from build123d import *

# Parameters (mm, degrees)
SKETCH1_R                          = 61.976
BOSS_EXTRUDE1_DEPTH                = 1.5875
F_1_4_0_25_DIAMETER_HOLE1_D        = 6.35
F_5_16_0_3125_DIAMETER_HOLE1_D     = 7.9375
F_5_16_0_3125_DIAMETER_HOLE1_DEPTH = 3.302


with BuildPart() as part:
    # Sketch1 → Boss-Extrude1 (new body, symmetric)
    with BuildSketch(Plane.XY):
        Circle(SKETCH1_R)
    extrude(amount=BOSS_EXTRUDE1_DEPTH, both=True)

    # 1/4 (0.25) Diameter Hole1 (through all)
    with Locations(Plane.XY.offset(1.5875)):
        with Locations((-47.625, 0), (47.625, 0)):
            Hole(F_1_4_0_25_DIAMETER_HOLE1_D / 2)

    # 5/16 (0.3125) Diameter Hole1
    with Locations(Plane.XY.offset(1.5875)):
        with Locations((0, 0)):
            Hole(F_5_16_0_3125_DIAMETER_HOLE1_D / 2, depth=F_5_16_0_3125_DIAMETER_HOLE1_DEPTH)


solid = part.part
Could you check a few things on this model? Use its own coordinates, in mm. Give positions to 0.01 mm unless a question says otherwise; leave off trailing zeros. Order: outer loops, then holes, each group sorted by start corner. A loop starts at its lowest first (then second) coordinate and runs counter-clockwise, first axis right, second up. Notation, with made-up numbers: (69, -38) -> (79, -38) arc R21 cw to (79, -30) -> close; hole circle Ø8 at (54, 50.5). An arc over 180 degrees is marked (long way). Answer in a Markdown table with one row per item. Add a question column.
Item 1: We'd pull the mould along Y, two halves only. Please class faces 1 (the cylindrical face through (33.318, 52.258, 0.022)), 2 (the cylindrical face through (0.86, -3.874, -0.022)), 3 (the flat face through (-1, -13, 1.588)): pulls with the +Y half, pulls with the -Y half, needs draft (parallel to the pull), parting line crosses it, or undercut.
Item 2: Please list where these lines run through material, in increasing order: probe 1 along Y at (x, z) = (0, 0.6); probe 2 along Y at (x, z) = (49, 1.35); probe 3 along Y at (x, z) = (55, 0.85).
Item 3: Imagine slicing it at D-D (x = 33). List the corners of the cut face in (y, z) for me, and give its area (3 significant figures).
Item 4: Imagine slicing it at C-C (z = 0.95). Count the separate pieces of the cut face and the enclosed holes in it, and give its area (3 significant figures).
Item 5: Imagine slicing it at B-B (y = 0). List the corners of the cut face in (x, z) for me.
Item 6: I'm going to push flat-ended pins straight in: P1, Ø1, axis at y = 7, z = 1, coming from the +X side; P2, Ø1, axis at x = -46.5, z = 1, coming from the -Y side; P3, Ø4, axis at x = -47.625, y = 0, coming from the +Z side (3 decimals); P4, Ø12.5, axis at x = 0, y = 0, coming from the +Z side. Where does each tip first touch, or does it pass through?
Item 7: Imagine slicing it at A-A (x = 0). List the corners of the cut face in (y, z) for me, and give its area (3 significant figures).
Result:
| question | item | result |
|---|---|---|
| 1 | face 1 | parting line crosses it |
| 1 | face 2 | undercut |
| 1 | face 3 | needs draft |
| 2 | probe 1 | -61.98 to -3.97, 3.97 to 61.98 |
| 2 | probe 2 | -37.95 to -2.86, 2.86 to 37.95 |
| 2 | probe 3 | -28.57 to 28.57 |
| 3 | outline | (-52.46, -1.59) -> (52.46, -1.59) -> (52.46, 1.59) -> (-52.46, 1.59) -> close |
| 3 | area | 333 mm2 |
| 4 | separate pieces | 1 |
| 4 | enclosed holes | 3 |
| 4 | area | 12,000 mm2 |
| 5 | outline | (-61.98, -1.59) -> (-50.8, -1.59) -> (-50.8, 1.59) -> (-61.98, 1.59) -> close; (-44.45, -1.59) -> (-3.97, -1.59) -> (-3.97, 1.59) -> (-44.45, 1.59) -> close; (3.97, -1.59) -> (44.45, -1.59) -> (44.45, 1.59) -> (3.97, 1.59) -> close; (50.8, -1.59) -> (61.98, -1.59) -> (61.98, 1.59) -> (50.8, 1.59) -> close |
| 6 | P1 | x = 61.63 |
| 6 | P2 | y = -41.53 |
| 6 | P3 | through |
| 6 | P4 | z = 1.59 |
| 7 | outline | (-61.98, -1.59) -> (-3.97, -1.59) -> (-3.97, 1.59) -> (-61.98, 1.59) -> close; (3.97, -1.59) -> (61.98, -1.59) -> (61.98, 1.59) -> (3.97, 1.59) -> close |
| 7 | area | 368 mm2 |
